Verification items for the finished model (mm, model axes). A direction names the side the tool comes from. Coordinates: 2 decimals unless noted, no trailing zeros. Loops run counter-clockwise (first coordinate to the right, second up) from the corner with the lowest first, then second, coordinate; pieces in that order, holes last. Notation, with made-up numbers: (-5, 25) -> (42, 25) arc R17 cw to (42, 52) -> close; hole circle Ø3 at (-35.5, 34). An arc over 180 degrees is marked (long way). Answer as a JSON object with one key per item and string values. Group by question number.
Q1. Cross-section at A-A on y = -11.75. Record the boundary of the cut face in (x, z).
Q2. Cross-section at B-B on z = -7.75. Record the boundary of the cut face in (x, y), and give its area (3 significant figures).
Q3. Release check for a two-part mould opening along X. For faces 3 (the flat face through (72.926, -12.522, -6.023)), 4 (the cylindrical face through (-49.19, -12.52, -13.37)), 5 (the flat face through (-1, 0, 1)) record: released by +X, released by -X, zero draft, split by the parting line, or undercut.
Q4. Cross-section at C-C on x = 7.5. Record the boundary of the cut face in (y, z).
Q5. Cross-section at D-D on z = 2.75. Record the boundary of the cut face in (x, y).
Q6. Set-up check for faces 1 (the flat face through (-20, -13, -18.392)), 2 (the flat face through (7, -13, 0)): record each of +Z, -Z, +X, -X, +Y, -Y from which the full face is reachable in a straight line by a thin tool's end or side.
Q7. Scan lines: L1, parallel to Z at x = 31, y = -23.5; L2, parallel to Z at x = -24.5, y = -16.75; L3, parallel to X at y = -3.5, z = 4. Record each from-to range of solid material in increasing order.
Q8. Gauge pin test, flat ends, axial feed: pin 1 Ø8 at (x, y) = (10, -20) entering from -Z; pin 2 Ø1 at (y, z) = (-22, 2.5) entering from +X; pin 3 Ø5 at (y, z) = (-11, -7.5) entering from +X (3 decimals). Record the tip position at first contact, or that the pin passes through.
```python
from build123d import *

# Parameters (mm, degrees)
F1_DEPTH = 25.4


# Not quite as in the source:
# - the program builds the solid bodies; features that only make, move or delete a surface that nothing else refers to are left out


with BuildPart() as f1:
    # F0 (on Front) → F1 (new body)
    with BuildSketch(Plane.XZ):
        with BuildLine():
            Line((-38.4986028075, 0), (54.1304424405, 0))
            Line((54.1304424405, 0), (92.2559946775, -12.2162923217))
            Line((92.2559946775, -12.2162923217), (54.1304424405, 8.1889424473))
            Line((54.1304424405, 8.1889424473), (-38.4986028075, 8.1889424473))
            ThreePointArc((-38.4986028075, 8.1889424473), (-49.8267048533, 5.777561047), (-59.1905941264, -1.0384666745))
            ThreePointArc((-59.1905941264, -1.0384666745), (-58.8832559342, -3.7017340098), (-58.2345825442, -6.3030168658))
            ThreePointArc((-58.2345825442, -6.3030168658), (-49.0469266103, -13.4580145444), (-38.4986028075, -18.3915607631))
            Line((-38.4986028075, -18.3915607631), (0, -18.3915607631))
            Line((0, -18.3915607631), (-38.4986028075, -12.2556750716))
            ThreePointArc((-38.4986028075, -12.2556750716), (-43.7271300367, -6.1278375358), (-38.4986028075, 0))
        make_face()
    extrude(amount=F1_DEPTH)


solid = f1.part
```
Computed values:
{
 "1": {"outline": "(-59.19, -1.04) arc R20.72 ccw to (-58.23, -6.3) arc R52.06 ccw to (-38.5, -18.39) -> (0, -18.39) -> (-38.5, -12.26) arc R6.21 cw to (-38.5, 0) -> (54.13, 0) -> (92.26, -12.22) -> (54.13, 8.19) -> (-38.5, 8.19) arc R27.81 ccw to start"},
 "2": {"outline": "(-56.69, -25.4) -> (-43.51, -25.4) -> (-43.51, 0) -> (-56.69, 0) -> close; (78.32, -25.4) -> (83.91, -25.4) -> (83.91, 0) -> (78.32, 0) -> close", "area": "477 mm²"},
 "3": {"face 3": "undercut", "face 4": "released by -X", "face 5": "zero draft"},
 "4": {"outline": "(-25.4, 0) -> (0, 0) -> (0, 8.19) -> (-25.4, 8.19) -> close"},
 "5": {"outline": "(-55.02, -25.4) -> (64.29, -25.4) -> (64.29, 0) -> (-55.02, 0) -> close"},
 "6": {"face 1": "-Z, +X, -X, +Y, -Y", "face 2": "+Y, -Y"},
 "7": {"L1": "z = 0 to 8.19", "L2": "z = -18.39 to -14.49, 0 to 8.19", "L3": "x = -53.18 to 61.96"},
 "8": {"pin 1": "stops at z = 0", "pin 2": "stops at x = 65.69", "pin 3": "stops at x = 88.115"}
}
